Check sheet for the modelled part. Datum: model origin and axes. Units: mm. Face numbers are marked on the shaded views. A direction names the side the tool comes from. Give positions to 0.01 mm unless a question says otherwise; leave off trailing zeros. Loops run counter-clockwise (first coordinate to the right, second up) from the corner with the lowest first, then second, coordinate; pieces in that order, holes last. Notation, with made-up numbers: M 25.25,-26.75 L 55.25,-26.75 A36 ccw 55.25,9.25 Z; hole C 48,39.25 d6. An arc over 180 degrees is marked long. Use one line per item in the form item = value.
Autodesk Inventor part; units mm, degrees
ref_plane "Tip Plane" through (-3.4636, -0.3407, 119.38) normal (0, 0, 1) x (1, 0, 0)
ref_plane "Clip" through (0, 4.0132, 0) normal (0, 1, 0) x (-1, 0, 0)
ref_plane "YZ Plane" through (0, 0, 0) normal (1, 0, 0) x (0, 1, 0)
sketch "Sketch1" plane through (0, 0, 0) normal (0, 0, 1) x (1, 0, 0)
  circle A0 centre (-3.4636, -0.3407) radius 4.445
  point P0 (0, 0)
  dimension "d0" = 8.89
extrude "Pen body" add sketch "Sketch1" along normal blind 101.6
ref_plane "Tip Plane" through (-3.4636, -0.3407, 119.38) normal (0, 0, 1) x (1, 0, 0)
sketch "Sketch2" plane through (-3.4636, -0.3407, 119.38) normal (0, 0, 1) x (1, 0, 0)
  circle A0 centre (0, 0) radius 0.0254
  point P0 (3.4636, 0.3407)
  dimension "d4" = 0.0508
loft "Body to Tip" add profiles "Sketch2" section 1 edges at (-7.9086, -0.3407, 101.6)
sketch "Sketch3" plane through (-3.4636, -0.3407, 0) normal (0, 0, -1) x (-1, 0, 0)
  point P0 (-3.4636, 0.3407)
sketch "Sketch4" plane through (-3.4636, -0.3407, 0) normal (0, 0, -1) x (-1, 0, 0)
  circle A0 centre (0, 0) radius 2.8396
  point P0 (-3.4636, 0.3407)
extrude "Click" add sketch "Sketch4" along normal blind 9.525
ref_plane "Clip" through (0, 4.0132, 0) normal (0, 1, 0) x (-1, 0, 0)
sketch "Clip extention" plane through (0, 4.0132, 0) normal (0, 1, 0) x (-1, 0, 0)
  point P0 (0, 0)
sketch "Clips extension's extension" plane through (0, 4.0132, 0) normal (0, 1, 0) x (-1, 0, 0)
  point P0 (0, 0)
sketch "Sketch7" plane through (0, 4.0132, 0) normal (0, 1, 0) x (-1, 0, 0)
  line L0 (4.5996, 1.2363) -> (2.3394, 1.2363)
  line L1 (2.3394, 1.2363) -> (2.3394, 2.4001)
  line L2 (2.3394, 2.4001) -> (4.5996, 2.4001)
  line L3 (4.5996, 2.4001) -> (4.5996, 1.2363)
  point P0 (0, 0)
extrude "Extrusion3" add sketch "Sketch7" along normal blind 2.032
sketch "Sketch8" plane through (-4.5996, 4.0132, 2.4001) normal (0, 0, 1) x (1, 0, 0)
  line L0 (0, 0) -> (0, 2.032)
  line L1 (2.2602, 0) -> (2.2602, 2.032)
  line L2 (0, 2.032) -> (2.2602, 2.032)
  line L3 (2.2602, 2.032) -> (2.2602, 1.1849)
  line L4 (2.2602, 1.1849) -> (0, 1.1849)
  line L5 (0, 1.1849) -> (0, 2.032)
  point P0 (4.5996, -4.0132)
extrude "Extrusion4" add sketch "Sketch8" along normal blind 21.082
properties part number "Pen"
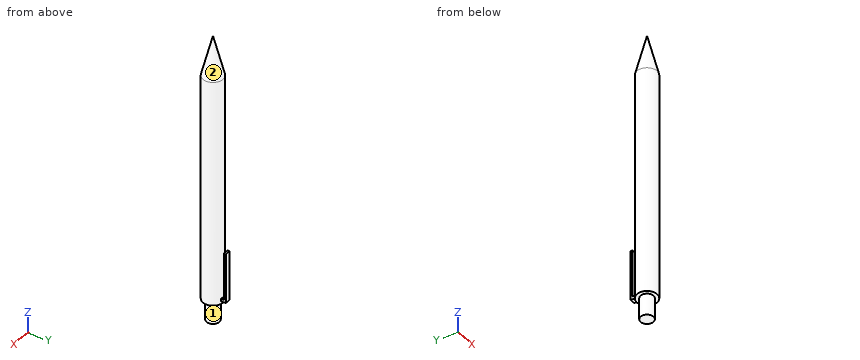
1) Set-up check for the marked faces 1 and 2: record each of +Z, -Z, +X, -X, +Y, -Y from which the full face is reachable in a straight line by a thin tool's end or side.
Evaluation:
face_1 = -Z
face_2 = +Z
2) Depth check by flat-ended pin: pin 1 Ø3 at (x, z) = (-1.5, 101.5) entering from +Y; pin 2 Ø0.9 at (x, y) = (-3, 5.5) entering from +Z; pin 3 Ø2 at (y, z) = (4.5, 14.5) entering from +X. Enter the tip coordinate at first touch or a pass-through.
Evaluation:
pin_1 = 4.08
pin_2 = 23.48
pin_3 = -1.23
3) Scan lines: line 1 (Z direction, x = -3.75, y = 5); line 2 (Y direction, x = -4.25, z = 9); line 3 (Y direction, x = -3.25, z = 57). Record each from-to range of solid material in increasing order.
Evaluation:
line_1 = 1.24 to 2.4
line_2 = -4.72 to 4.03, 5.2 to 6.05
line_3 = -4.78 to 4.1
4) Section check A-A (z = 31). Record the cut outline in (x, y) (3 decimals), then the cut area to 3 significant figures.
Evaluation:
outline = C -3.464,-0.341 d8.89
area = 62.1 mm^2
5) Section check B-B (z = 104). Record the cut outline in (x, y).
Evaluation:
outline = C -3.46,-0.34 d7.7
